Check sheet for the modelled part. Datum: model origin and axes. Units: mm. Face numbers are marked on the shaded views. A direction names the side the tool comes from. Round coordinates to 2 decimals unless told otherwise and drop trailing zeros. Loops run counter-clockwise (first coordinate to the right, second up) from the corner with the lowest first, then second, coordinate; pieces in that order, holes last. Notation, with made-up numbers: (19, 55) - (35, 55) arc R7 cw to (35, 68) - close; hole circle Ø8 at (74, 23.5). An arc over 180 degrees is marked (long way). Put each result on its own line as item: value.
```python
from build123d import *

# Parameters (mm, degrees)
BOSS_EXTRUDE1_START      = 3.6
SKETCH2_W                = 22
SKETCH2_H                = 28
SKETCH2_W_2              = 18
SKETCH2_H_2              = 12
SKETCH2_W_3              = 4.5
SKETCH2_H_3              = 5
SKETCH2_W_4              = 17
BOSS_EXTRUDE1_DEPTH      = 5
SKETCH2_3_W              = 17
SKETCH2_3_H              = 5
BOSS_EXTRUDE2_DEPTH      = 8.6
SKETCH2_7_W              = 17
SKETCH2_7_H              = 18.5
BOSS_EXTRUDE3_DEPTH      = 8.6
M3_CLEARANCE_HOLE1_D     = 3.2
M3_CLEARANCE_HOLE1_DEPTH = 5
M3_CLEARANCE_HOLE1_TIP   = 0.96137699
FILLET1_R                = 1


with BuildPart() as part:
    # Sketch2 → Boss-Extrude1 (new body)
    # profile 1 of 5: a face of its own
    with BuildSketch(Plane(origin=(0, 0, 0), x_dir=(0, 0, -1), z_dir=(1, 0, 0)).offset(BOSS_EXTRUDE1_START)):
        Polygon((-13, 22.5), (-8.5, 22.5), (8.5, 22.5), (13, 22.5), (13, -8.5), (-13, -8.5), align=None)
        with Locations((0, 6.5)):
            Rectangle(SKETCH2_W, SKETCH2_H, mode=Mode.SUBTRACT)
    # profile 2 of 5: a face of its own
    with BuildSketch(Plane(origin=(0, 0, 0), x_dir=(0, 0, -1), z_dir=(1, 0, 0)).offset(BOSS_EXTRUDE1_START)):
        with Locations((0, 6.5)):
            Rectangle(SKETCH2_W, SKETCH2_H)
        with Locations((0, 13.5)):
            Rectangle(SKETCH2_W_2, SKETCH2_H_2, mode=Mode.SUBTRACT)
    # profile 3 of 5: a face of its own
    with BuildSketch(Plane(origin=(0, 0, 0), x_dir=(0, 0, -1), z_dir=(1, 0, 0)).offset(BOSS_EXTRUDE1_START)):
        with Locations((10.75, 25)):
            Rectangle(SKETCH2_W_3, SKETCH2_H_3)
    # profile 4 of 5: a face of its own
    with BuildSketch(Plane(origin=(0, 0, 0), x_dir=(0, 0, -1), z_dir=(1, 0, 0)).offset(BOSS_EXTRUDE1_START)):
        with Locations((0, 25)):
            Rectangle(SKETCH2_W_4, SKETCH2_H_3)
    # profile 5 of 5: a face of its own
    with BuildSketch(Plane(origin=(0, 0, 0), x_dir=(0, 0, -1), z_dir=(1, 0, 0)).offset(BOSS_EXTRUDE1_START)):
        with Locations((-10.75, 25)):
            Rectangle(SKETCH2_W_3, SKETCH2_H_3)
    extrude(amount=BOSS_EXTRUDE1_DEPTH)

    # Sketch2<3> → Boss-Extrude2 (add)
    with BuildSketch(Plane(origin=(0, 0, 0), x_dir=(0, 0, -1), z_dir=(1, 0, 0))):
        with Locations((0, 25)):
            Rectangle(SKETCH2_3_W, SKETCH2_3_H)
    extrude(amount=BOSS_EXTRUDE2_DEPTH)

    # Sketch2<7> → Boss-Extrude3 (add)
    with BuildSketch(Plane(origin=(0, 0, 0), x_dir=(0, 0, -1), z_dir=(1, 0, 0))):
        with Locations((0, 36.75)):
            Rectangle(SKETCH2_7_W, SKETCH2_7_H)
        with BuildLine():
            Line((3, 28), (-3, 28))
            ThreePointArc((-3, 28), (-7, 32), (-3, 36))
            Line((-3, 36), (3, 36))
            ThreePointArc((3, 36), (7, 32), (3, 28))
        make_face(mode=Mode.SUBTRACT)
    extrude(amount=BOSS_EXTRUDE3_DEPTH)

    # M3 Clearance Hole1
    with Locations(Plane(origin=(8.6, 0, 0), x_dir=(0, 0, -1), z_dir=(1, 0, 0))):
        with Locations((-5, 41), (5, 41)):
            Hole(M3_CLEARANCE_HOLE1_D / 2, depth=M3_CLEARANCE_HOLE1_DEPTH)
            with Locations((0, 0, -(M3_CLEARANCE_HOLE1_DEPTH + M3_CLEARANCE_HOLE1_TIP / 2))):  # 118° drill point
                Cone(0, M3_CLEARANCE_HOLE1_D / 2, M3_CLEARANCE_HOLE1_TIP, mode=Mode.SUBTRACT)

    # Fillet1
    fillet1_edges = [part.edges().sort_by_distance(p)[0] for p in [
        (1.8, 22.5, 8.5),
        (1.8, 22.5, -8.5),
        (4.3, 46, -8.5),
        (4.3, 46, 8.5),
    ]]
    fillet(fillet1_edges, radius=FILLET1_R)


solid = part.part
```
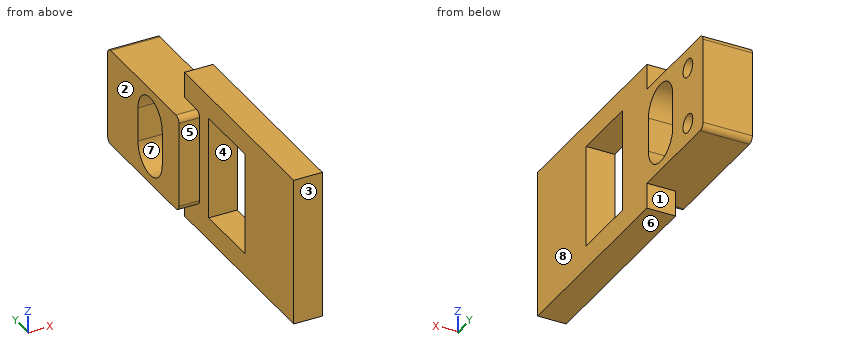
Item 1: Release check for a two-part mould opening along Z. For the marked faces 6, 7 and 8 record: +Z half, -Z half, draft (parallel to the pull), parting line (faces both ways), or undercut.
Filled sheet:
face 6: -Z half
face 7: undercut
face 8: draft
Item 2: Section check C-C on x = 7. Enter the section's corners in (y, z).
Filled sheet:
outline: (-8.5, -13) - (27.5, -13) - (27.5, -8.5) - (45, -8.5) arc R1 ccw to (46, -7.5) - (46, 7.5) arc R1 ccw to (45, 8.5) - (27.5, 8.5) - (27.5, 13) - (-8.5, 13) - close; hole (7.5, -9) - (19.5, -9) - (19.5, 9) - (7.5, 9) - close; hole (28, -3) arc R4 ccw to (36, -3) - (36, 3) arc R4 ccw to (28, 3) - close; hole circle Ø3.2 at (41, -5); hole circle Ø3.2 at (41, 5)
Item 3: Section check B-B on z = 2.25. Enter the section's corners in (x, y).
Filled sheet:
outline: (0, 22.5) - (3.6, 22.5) - (3.6, 19.5) - (8.6, 19.5) - (8.6, 28) - (0, 28) - close; (0, 36) - (8.6, 36) - (8.6, 46) - (0, 46) - close; (3.6, -8.5) - (8.6, -8.5) - (8.6, 7.5) - (3.6, 7.5) - close
Item 4: Thickness scan on line 1 (Z direction, x = 5.2, y = 41); line 2 (Y direction, x = 4.75, z = -3.25); line 3 (Z direction, x = 6, y = 17.5). Record the ranges inside material, lowest first. Write a range as from..to.
Filled sheet:
line 1: -8.5..-6.6, -3.4..3.4, 6.6..8.5
line 2: -8.5..7.5, 19.5..28.01, 35.99..46
line 3: -13..-9, 9..13
Item 5: Section check A-A on y = 8. Enter the section's corners in (x, z), then the cut area to 3 significant figures.
Filled sheet:
outline: (3.6, -13) - (8.6, -13) - (8.6, -9) - (3.6, -9) - close; (3.6, 9) - (8.6, 9) - (8.6, 13) - (3.6, 13) - close
area: 40.0 mm²
Item 6: Section check D-D on x = 0.5. Enter the section's corners in (y, z).
Filled sheet:
outline: (22.5, -7.5) arc R1 ccw to (23.5, -8.5) - (45, -8.5) arc R1 ccw to (46, -7.5) - (46, 7.5) arc R1 ccw to (45, 8.5) - (23.5, 8.5) arc R1 ccw to (22.5, 7.5) - close; hole (28, -3) arc R4 ccw to (36, -3) - (36, 3) arc R4 ccw to (28, 3) - close
Item 7: Tool access check on the marked faces 1, 2, 3, 4 and 5. Record the directions out of +Z, -Z, +X, -X, +Y, -Y that give a thin tool (end or side, any length) a straight path to the whole face; none if there is none.
Filled sheet:
face 1: -Z, +X, -X, +Y
face 2: +Z, -Z, -X, +Y, -Y
face 3: +Z, -Z, +X, -X, -Y
face 4: +X, -X
face 5: +Z, -Z, -X, -Y
Item 8: Go/stop test with flat-tipped pins: pin 1 (5 mm diameter, centred on x = 6.5, z = -11.5, fed in from +Y); pin 2 (3 mm diameter, centred on y = 41, z = -5, fed in from +X); pin 3 (2.5 mm diameter, centred on x = 3.5, y = 31.5, fed in from +Z). Record where each tip stops, or that it passes through.
Filled sheet:
pin 1: y = 27.5
pin 2: x = 3.54
pin 3: z = 8.5
